Geometry: final body of the model. Coordinates: model frame, mm. Face numbers are marked on the shaded views. A direction names the side the tool comes from. Round coordinates to 2 decimals unless told otherwise and drop trailing zeros. Loops run counter-clockwise (first coordinate to the right, second up) from the corner with the lowest first, then second, coordinate; pieces in that order, holes last. Notation, with made-up numbers: M -13.75,-19 L 21.25,-19 A30 ccw 21.25,5 Z; hole C 84,84 d3. An arc over 180 degrees is marked long. Return JSON: item names as keys, results as strings.
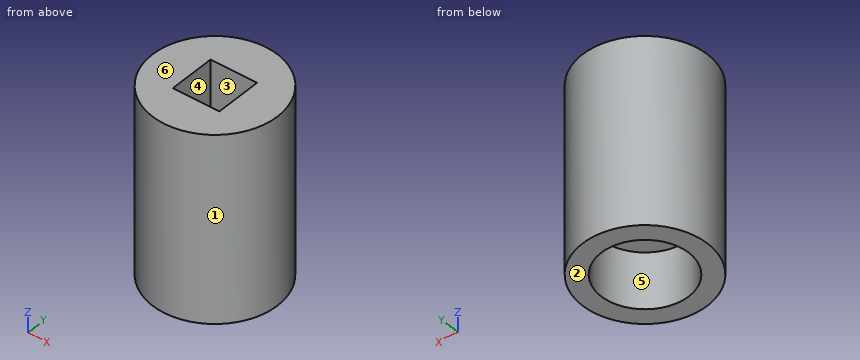
from build123d import *

# Parameters (mm, degrees)
SKETCH1_R           = 3.35
BOSS_EXTRUDE1_DEPTH = 10
SKETCH2_W           = 2.5
SKETCH2_H           = 2.5
CUT_EXTRUDE1_DEPTH  = 5
SKETCH3_R           = 2.35
CUT_EXTRUDE2_DEPTH  = 3
SKETCH4_R           = 1
CUT_EXTRUDE3_DEPTH  = 3


with BuildPart() as part:
    # Sketch1 → Boss-Extrude1 (new body)
    with BuildSketch(Plane.XY):
        Circle(SKETCH1_R)
    extrude(amount=BOSS_EXTRUDE1_DEPTH)

    # Sketch2 → Cut-Extrude1 (cut)
    with BuildSketch(Plane.XY.offset(10)):
        Rectangle(SKETCH2_W, SKETCH2_H)
    extrude(amount=-CUT_EXTRUDE1_DEPTH, mode=Mode.SUBTRACT)

    # Sketch3 → Cut-Extrude2 (cut)
    with BuildSketch(Plane(origin=(0, 0, 0), x_dir=(-1, 0, 0), z_dir=(0, 0, -1))):
        Circle(SKETCH3_R)
    extrude(amount=-CUT_EXTRUDE2_DEPTH, mode=Mode.SUBTRACT)

    # Sketch4 → Cut-Extrude3 (cut)
    with BuildSketch(Plane(origin=(0, 0, 3), x_dir=(-1, 0, 0), z_dir=(0, 0, -1))):
        Circle(SKETCH4_R)
    extrude(amount=-CUT_EXTRUDE3_DEPTH, mode=Mode.SUBTRACT)


solid = part.part
Q1. Section query A-A (y = 0). Output: boundary loops of the cut face in (x, z), plus the area to 3 significant figures.
Determined:
{"outline": "M -3.35,0 L -2.35,0 L -2.35,3 L -1,3 L -1,5 L -1.25,5 L -1.25,10 L -3.35,10 Z; M 1,3 L 2.35,3 L 2.35,0 L 3.35,0 L 3.35,10 L 1.25,10 L 1.25,5 L 1,5 Z", "area": "36.4 mm^2"}
Q2. Section query C-C (z = 8.5). Output: boundary loops of the cut face in (x, y), plus the area to 3 significant figures.
Determined:
{"outline": "C 0,0 d6.7; hole M -1.25,-1.25 L 1.25,-1.25 L 1.25,1.25 L -1.25,1.25 Z", "area": "29.0 mm^2"}
Q3. Pin query (flat end, axial travel): pin 1 (3 mm diameter, centred on x = 0, y = 0, fed in from -Z); pin 2 (1 mm diameter, centred on x = -2.5, z = 6, fed in from +Y). Return the tip coordinate at first contact, or that it passes through.
Determined:
{"pin 1": "stops at z = 3", "pin 2": "stops at y = 2.69"}
Q4. Reachability of the marked faces 4, 5 and 6 from +Z, -Z, +X, -X, +Y, -Y: full face, straight path, thin tool, end or side. Return the list, or none.
Determined:
{"face 4": "+Z", "face 5": "-Z", "face 6": "+Z, +X, -X, +Y, -Y"}
Q5. Section query D-D (x = 1.5). Output: boundary loops of the cut face in (y, z), plus the area to 3 significant figures.
Determined:
{"outline": "M -3,0 L -1.81,0 L -1.81,3 L 1.81,3 L 1.81,0 L 3,0 L 3,10 L -3,10 Z", "area": "49.1 mm^2"}
Q6. Pull-direction query (X, two-part tool) for the marked faces 1, 2 and 3; classes: pulls with the +X half, pulls with the -X half, needs draft (parallel to the pull), parting line crosses it, or undercut.
Determined:
{"face 1": "parting line crosses it", "face 2": "needs draft", "face 3": "undercut"}
Q7. Material intervals for L1, parallel to Y at x = 0, z = 2.25; L2, parallel to Y at x = 0, z = 4.6; L3, parallel to X at y = 0.75, z = 9, sorted ascending.
Determined:
{"L1": "y = -3.35 to -2.35, 2.35 to 3.35", "L2": "y = -3.35 to -1, 1 to 3.35", "L3": "x = -3.26 to -1.25, 1.25 to 3.26"}
